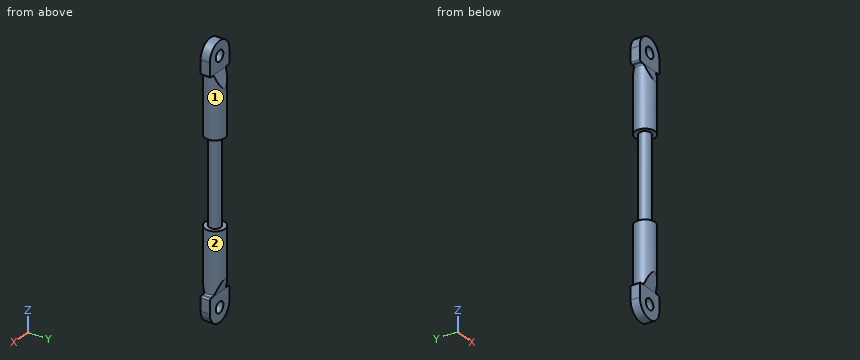
```python
from build123d import *

# Parameters (mm, degrees)
SKETCH1_R                  = 2
SCREW_SECTION_DEPTH        = 15
SKETCH2_R                  = 3.5
BAR_SECTION_DEPTH          = 21.5
MOUNT_SECTION_DEPTH        = 1.6
BAR_TAPER_DEPTH            = 6
MOUNT_FILLET_R             = 0.5
MOUNT_FILLET_OF_MIRROR_2_R = 0.5


with BuildPart() as part:
    # Sketch1 → Screw Section (new body)
    with BuildSketch(Plane.XY):
        Circle(SKETCH1_R)
    screw_section = extrude(amount=SCREW_SECTION_DEPTH)

    # Sketch2 → Bar Section (add)
    with BuildSketch(Plane.XY.offset(15)):
        Circle(SKETCH2_R)
    bar_section = extrude(amount=BAR_SECTION_DEPTH)

    # Sketch3 → Mount Section (add, symmetric)
    with BuildSketch(Plane(origin=(0, 0, 0), x_dir=(1, 0, 0), z_dir=(0, 1, 0))):
        with BuildLine():
            Line((5, -36.5), (-5, -36.5))
            Line((-5, -36.5), (-5, -41.5))
            ThreePointArc((-5, -41.5), (0, -46.5), (5, -41.5))
            Line((5, -41.5), (5, -36.5))
        make_face()
    mount_section = extrude(amount=MOUNT_SECTION_DEPTH, both=True)

    # Sketch4 → Bar Taper (cut, symmetric)
    with BuildSketch(Plane(origin=(0, 0, 0), x_dir=(0, 0, -1), z_dir=(1, 0, 0))):
        Polygon((-31.5, -3.5), (-36.5, -1.6), (-36.5, -3.5), align=None)
        Polygon((-31.5, 3.5), (-36.5, 1.6), (-36.5, 3.5), align=None)
    bar_taper = extrude(amount=BAR_TAPER_DEPTH, both=True, mode=Mode.SUBTRACT)

    # Mount Fillet
    mount_fillet_edges = [part.edges().sort_by_distance(p)[0] for p in [
        (-5, 0, 36.5),
        (3.401842713, -0.823083322, 36.5),
        (-3.5, 0, 36.5),
        (5, 0, 36.5),
    ]]
    fillet(mount_fillet_edges, radius=MOUNT_FILLET_R)

    # Sketch6 → Ball Hole (revolve, cut)
    with BuildSketch(Plane(origin=(0, 0, 0), x_dir=(0, 0, -1), z_dir=(1, 0, 0))):
        with BuildLine():
            Line((-43.420937271, -1.6), (-41.5, -1.6))
            Line((-41.5, -1.6), (-41.5, 1.6))
            Line((-41.5, 1.6), (-43.420937271, 1.6))
            ThreePointArc((-43.420937271, 1.6), (-44, 0), (-43.420937271, -1.6))
        make_face()
    ball_hole = revolve(axis=Axis((0, -1.6, 41.5), (0, 1, 0)), mode=Mode.SUBTRACT)

    # Mirror 2: Screw Section, Bar Section, Mount Section, Bar Taper, Ball Hole across Front Plane
    add(screw_section.mirror(Plane.XY))
    add(bar_section.mirror(Plane.XY))
    add(mount_section.mirror(Plane.XY))
    add(bar_taper.mirror(Plane.XY), mode=Mode.SUBTRACT)
    add(ball_hole.mirror(Plane.XY), mode=Mode.SUBTRACT)

    # Mount Fillet of Mirror 2
    mount_fillet_of_mirror_2_edges = [part.edges().sort_by_distance(p)[0] for p in [
        (-5, 0, -36.5),
        (3.401842713, -0.823083322, -36.5),
        (-3.5, 0, -36.5),
        (5, 0, -36.5),
    ]]
    fillet(mount_fillet_of_mirror_2_edges, radius=MOUNT_FILLET_OF_MIRROR_2_R)


solid = part.part
```
Source: CAD feature listing. Evaluate the final solid. Frame: model axes, mm. Face numbers are marked on the shaded views. Give positions to 0.01 mm unless a question says otherwise; leave off trailing zeros. Loops run counter-clockwise (first coordinate to the right, second up) from the corner with the lowest first, then second, coordinate; pieces in that order, holes last. Notation, with made-up numbers: (66, 6.5) -> (123, 6.5) arc R28 ccw to (123, 43.5) -> close; hole circle Ø11 at (1, 12). An arc over 180 degrees is marked (long way). Use a Markdown table: item, result. Add a question column.
(1) Section query A-A (y = 0). Count the separate pieces of the cut face and the enclosed holes in it, then the cut area to 3 significant figures.
(2) Ray query, line 1 (Z direction, x = 0.25, y = -0.5); line 2 (Y direction, x = -3.25, z = 40); line 3 (Z direction, x = 3.75, y = 0.75). Return the intervals inside material, ascending.
(3) Pull-direction query (Z, two-part tool) for the marked faces 1 and 2; classes: +Z half, -Z half, draft (parallel to the pull), parting line (faces both ways), or undercut.
(4) Section query B-B (x = 0). Output: boundary loops of the cut face in (y, z), then the cut area to 3 significant figures.
(5) First-contact query: pin 1 Ø5 at (x, z) = (2.5, -40) entering from -Y; pin 2 Ø3 at (y, z) = (2, 12) entering from +X; pin 3 Ø3.5 at (x, y) = (1.5, 0) entering from -Z; pin 4 Ø3 at (x, z) = (-0.5, 40) entering from +Y. Flat tips, straight axial feed; report the tip coordinate or a pass-through.
(6) Section query C-C (z = 2.5). Output: boundary loops of the cut face in (x, y).
Checked values:
| question | item | result |
|---|---|---|
| 1 | separate pieces | 1 |
| 1 | enclosed holes | 2 |
| 1 | area | 560 mm^2 |
| 2 | line 1 | -46.49 to -43.94, -39.06 to 39.06, 43.94 to 46.49 |
| 2 | line 2 | -1.6 to 1.6 |
| 2 | line 3 | -44.81 to -36.47, 36.47 to 44.81 |
| 3 | face 1 | undercut |
| 3 | face 2 | undercut |
| 4 | outline | (-3.5, -31.5) -> (-1.6, -36.5) -> (-1.6, -39.58) arc R2.5 cw to (1.6, -39.58) -> (1.6, -36.5) -> (3.5, -31.5) -> (3.5, -15) -> (2, -15) -> (2, 15) -> (3.5, 15) -> (3.5, 31.5) -> (1.6, 36.5) -> (1.6, 39.58) arc R2.5 cw to (-1.6, 39.58) -> (-1.6, 36.5) -> (-3.5, 31.5) -> (-3.5, 15) -> (-2, 15) -> (-2, -15) -> (-3.5, -15) -> close; (-1.6, -46.5) -> (1.6, -46.5) -> (1.6, -43.42) arc R2.5 cw to (-1.6, -43.42) -> close; (-1.6, 43.42) arc R2.5 cw to (1.6, 43.42) -> (1.6, 46.5) -> (-1.6, 46.5) -> close |
| 4 | area | 436 mm^2 |
| 5 | pin 1 | y = -1.6 |
| 5 | pin 2 | x = 1.94 |
| 5 | pin 3 | z = -46.5 |
| 5 | pin 4 | y = 1.6 |
| 6 | outline | circle Ø4 at (0, 0) |
